```python
from build123d import *

# Parameters (mm, degrees)
SKETCH1_W           = 160
SKETCH1_H           = 55
BOSS_EXTRUDE1_DEPTH = 3.75
SKETCH2_W           = 14
SKETCH2_H           = 14
CUT_EXTRUDE1_DEPTH  = 3.5


with BuildPart() as part:
    # Sketch1 → Boss-Extrude1 (new, symmetric)
    with BuildSketch(Plane(origin=(0, 0, 0), x_dir=(1, 0, 0), z_dir=(0, 1, 0))):
        Rectangle(SKETCH1_W, SKETCH1_H)
    extrude(amount=BOSS_EXTRUDE1_DEPTH, both=True)

    # Sketch2 → Cut-Extrude1 (cut)
    with BuildSketch(Plane.XZ.offset(3.75)):
        with Locations((69.168154724, 17.5)):
            Rectangle(SKETCH2_W, SKETCH2_H)
        with Locations((69.168154724, -17.5)):
            Rectangle(SKETCH2_W, SKETCH2_H)
        Polygon((-41.168154724, -9.5), (-31.168154724, -9.5), (-31.168154724, -25.5), (-77.168154724, -25.5), (-77.168154724, 25.5), (-31.168154724, 25.5), (-31.168154724, 9.5), (-41.168154724, 9.5), align=None)
    extrude(amount=-CUT_EXTRUDE1_DEPTH, mode=Mode.SUBTRACT)


solid = part.part
```
For this review, take the finished solid that the model builds, in its own axes (mm). A direction names the side the tool comes from. Coordinates: 2 decimals unless noted, no trailing zeros. Loops run counter-clockwise (first coordinate to the right, second up) from the corner with the lowest first, then second, coordinate; pieces in that order, holes last.
1. Mouldability with a two-part tool opening along X and no side actions: class faces 3 (the flat face through (-36, -2, -9.5)), 4 (the flat face through (-1, 3.75, 0)), 5 (the flat face through (-36, -2, 9.5)), 6 (the flat face through (-80, 0, 0)) as +X half, -X half, draft (parallel to the pull), parting line (faces both ways), or undercut.
2. Add section B-B, the plane z = 23. Give the boundary of the cut face in (x, y), then the cut area to 3 significant figures.
3. Insertion check: P1, Ø4, axis at x = 66.5, z = 17.5, coming from the -Y side. The pin has a flat end and moves straight along its axis. Give the tip position at first contact, or say it passes through.
4. For faces 1 (the flat face through (69, -2, 24.5)), 2 (the flat face through (-1, 0, 27.5)), list the 3-axis set-ups (+Z, -Z, +X, -X, +Y, -Y) from which the entire face can be reached by the end or side of a thin tool; tool diameter is ignored.
5. For line 1 (X direction, y = -3, z = -23); line 2 (Y direction, x = -35, z = 15.5); line 3 (X direction, y = -2.75, z = -10), list the stretches that pass through material, from the lowest coordinate up.
6. Add section A-A, the plane x = -44.5. Give the boundary of the cut face in (y, z).
Result:
1. face 3: undercut
1. face 4: draft
1. face 5: undercut
1. face 6: -X half
2. outline: (-80, -3.75) - (-77.17, -3.75) - (-77.17, -0.25) - (-31.17, -0.25) - (-31.17, -3.75) - (62.17, -3.75) - (62.17, -0.25) - (76.17, -0.25) - (76.17, -3.75) - (80, -3.75) - (80, 3.75) - (-80, 3.75) - close
2. area: 990 mm2
3. P1: stops at y = -0.25
4. face 1: -Y
4. face 2: +Z, +X, -X, +Y, -Y
5. line 1: x = -80 to -77.17, -31.17 to 62.17, 76.17 to 80
5. line 2: y = -0.25 to 3.75
5. line 3: x = -80 to -77.17, -31.17 to 80
6. outline: (-3.75, -27.5) - (3.75, -27.5) - (3.75, 27.5) - (-3.75, 27.5) - (-3.75, 25.5) - (-0.25, 25.5) - (-0.25, -25.5) - (-3.75, -25.5) - close
